from build123d import *

# Parameters (mm, degrees)
SKETCH1_W           = 22
SKETCH1_H           = 31.5
BOSS_EXTRUDE1_DEPTH = 20
SKETCH2_R           = 5.4
CUT_EXTRUDE1_DEPTH  = 20
SKETCH3_R           = 1.5
CUT_EXTRUDE2_DEPTH  = 20
SKETCH4_W           = 22
SKETCH4_H           = 20
SKETCH4_R           = 1.5
BOSS_EXTRUDE2_DEPTH = 0.4
SKETCH5_R           = 44.087047381
CUT_EXTRUDE3_DEPTH  = 0.4
FILLET2_R           = 1
SKETCH6_R           = 1.6
BOSS_EXTRUDE3_DEPTH = 2


with BuildPart() as part:
    # Sketch1 → Boss-Extrude1 (new body)
    with BuildSketch(Plane.XY):
        Polygon((22, 2), (24, 2), (24, -33.5), (-2, -33.5), (-2, 2), align=None)
        with Locations((11, -15.75)):
            Rectangle(SKETCH1_W, SKETCH1_H, mode=Mode.SUBTRACT)
    extrude(amount=BOSS_EXTRUDE1_DEPTH)

    # Sketch2 → Cut-Extrude1 (cut)
    with BuildSketch(Plane(origin=(0, 2, 0), x_dir=(1, 0, 0), z_dir=(0, 1, 0))):
        with Locations((11, -10)):
            Circle(SKETCH2_R)
    extrude(amount=-CUT_EXTRUDE1_DEPTH, mode=Mode.SUBTRACT)

    # Sketch3 → Cut-Extrude2 (cut)
    with BuildSketch(Plane(origin=(0, -33.5, 0), x_dir=(-1, 0, 0), z_dir=(0, -1, 0))):
        with Locations((-11, -10)):
            Circle(SKETCH3_R)
    extrude(amount=-CUT_EXTRUDE2_DEPTH, mode=Mode.SUBTRACT)

    # Sketch4 → Boss-Extrude2 (add)
    with BuildSketch(Plane(origin=(0, -31.5, 0), x_dir=(1, 0, 0), z_dir=(0, 1, 0))):
        with Locations((11, -10)):
            Rectangle(SKETCH4_W, SKETCH4_H)
        with Locations((11, -10)):
            Circle(SKETCH4_R, mode=Mode.SUBTRACT)
    extrude(amount=BOSS_EXTRUDE2_DEPTH)

    # Sketch5 → Cut-Extrude3 (cut)
    with BuildSketch(Plane(origin=(0, -33.5, 0), x_dir=(-1, 0, 0), z_dir=(0, -1, 0))):
        with Locations((-11, -10)):
            Circle(SKETCH5_R)
    extrude(amount=-CUT_EXTRUDE3_DEPTH, mode=Mode.SUBTRACT)

    # Fillet2
    fillet2_edges = [part.edges().sort_by_distance(p)[0] for p in [
        (24, -33.1, 10),
        (-2, -33.1, 10),
        (-2, 2, 10),
        (24, 2, 10),
    ]]
    fillet(fillet2_edges, radius=FILLET2_R)

    # Sketch6 → Boss-Extrude3 (add)
    with BuildSketch(Plane.XY.offset(20)):
        with BuildLine():
            Line((22, -31.1), (27, -31.1))
            ThreePointArc((27, -31.1), (31, -27.1), (27, -23.1))
            Line((27, -23.1), (22, -23.1))
            Line((22, -23.1), (22, -31.1))
        make_face()
        with Locations((27, -27.1)):
            Circle(SKETCH6_R, mode=Mode.SUBTRACT)
        with BuildLine():
            Line((27, -11.1), (22, -11.1))
            Line((22, -11.1), (22, -3.1))
            Line((22, -3.1), (27, -3.1))
            ThreePointArc((27, -3.1), (31, -7.1), (27, -11.1))
        make_face()
        with Locations((27, -7.1)):
            Circle(SKETCH6_R, mode=Mode.SUBTRACT)
        with BuildLine():
            Line((0, -3.1), (-5, -3.1))
            ThreePointArc((-5, -3.1), (-9, -7.1), (-5, -11.1))
            Line((-5, -11.1), (0, -11.1))
            Line((0, -11.1), (0, -3.1))
        make_face()
        with Locations((-5, -7.1)):
            Circle(SKETCH6_R, mode=Mode.SUBTRACT)
        with BuildLine():
            Line((0, -23.1), (0, -31.1))
            Line((0, -31.1), (-5, -31.1))
            ThreePointArc((-5, -31.1), (-9, -27.1), (-5, -23.1))
            Line((-5, -23.1), (0, -23.1))
        make_face()
        with Locations((-5, -27.1)):
            Circle(SKETCH6_R, mode=Mode.SUBTRACT)
    extrude(amount=-BOSS_EXTRUDE3_DEPTH)


solid = part.part
Geometry check sheet. Reference: the model listing, model coordinates, mm. A direction names the side the tool comes from. Give positions to 0.01 mm unless a question says otherwise; leave off trailing zeros. Order: outer loops, then holes, each group sorted by start corner. A loop starts at its lowest first (then second) coordinate and runs counter-clockwise, first axis right, second up.
1) Cross-section at A-A (y = -15.5). Record the boundary of the cut face in (x, z), then the cut area to 3 significant figures.
Results are:
outline: (-2, 0) - (0, 0) - (0, 20) - (-2, 20) - close; (22, 0) - (24, 0) - (24, 20) - (22, 20) - close
area: 80.0 mm2
2) Tool access check on faces 4 (the flat face through (-4, -11.1, 19)), 5 (the flat face through (25, -3.1, 19)), 6 (the flat face through (-6, -5, 18)). Record the directions out of +Z, -Z, +X, -X, +Y, -Y that give a thin tool (end or side, any length) a straight path to the whole face; none if there is none.
Results are:
face 4: +Z, -Z, -X
face 5: +Z, -Z, +X, +Y
face 6: -Z, -X, +Y, -Y
3) Gauge pin test, flat ends, axial feed: pin 1 (1.6 mm diameter, centred on x = -3.5, z = 19, fed in from -Y); pin 2 (12 mm diameter, centred on x = 25, z = 15, fed in from -Y); pin 3 (5.5 mm diameter, centred on x = -7, y = -8, fed in from -Z); pin 4 (12 mm diameter, centred on x = 9.5, y = -16, fed in from -Z). Record the tip position at first contact, or that the pin passes through.
Results are:
pin 1: stops at y = -31.1
pin 2: stops at y = -33.1
pin 3: stops at z = 18
pin 4: passes through
4) Cross-section at D-D (x = 13.5). Record the boundary of the cut face in (y, z), then the cut area to 3 significant figures.
Results are:
outline: (-33.1, 0) - (-31.1, 0) - (-31.1, 20) - (-33.1, 20) - close; (0, 0) - (2, 0) - (2, 5.21) - (0, 5.21) - close; (0, 14.79) - (2, 14.79) - (2, 20) - (0, 20) - close
area: 60.9 mm2
5) Cross-section at B-B (z = 10). Record the boundary of the cut face in (x, y), then the cut area to 3 significant figures.
Results are:
outline: (-2, -32.1) arc R1 ccw to (-1, -33.1) - (9.5, -33.1) - (9.5, -31.1) - (0, -31.1) - (0, 0) - (5.6, 0) - (5.6, 2) - (-1, 2) arc R1 ccw to (-2, 1) - close; (12.5, -33.1) - (23, -33.1) arc R1 ccw to (24, -32.1) - (24, 1) arc R1 ccw to (23, 2) - (16.4, 2) - (16.4, 0) - (22, 0) - (22, -31.1) - (12.5, -31.1) - close
area: 200 mm2
6) Draft check along Y on faces 1 (the cylindrical face through (10.901, -32.114, 8.503)), 2 (the cylindrical face through (-5.35, -28.66, 19.01)), 3 (the cylindrical face through (-1.715, -32.799, 10.14)). Enter one of: released by +Y, released by -Y, zero draft, split by the parting line, or undercut.
Results are:
face 1: zero draft
face 2: undercut
face 3: released by -Y
7) Cross-section at C-C (y = -7.1). Record the boundary of the cut face in (x, z).
Results are:
outline: (-9, 18) - (-6.6, 18) - (-6.6, 20) - (-9, 20) - close; (-3.4, 18) - (-2, 18) - (-2, 0) - (0, 0) - (0, 20) - (-3.4, 20) - close; (22, 0) - (24, 0) - (24, 18) - (25.4, 18) - (25.4, 20) - (22, 20) - close; (28.6, 18) - (31, 18) - (31, 20) - (28.6, 20) - close
8) Material ranges on probe 1 along Y at (x, z) = (-5, 18.55); probe 2 along X at (y, z) = (-23, 17); probe 3 along Y at (x, z) = (0.5, 3.5), recorded low to high.
Results are:
probe 1: y = -31.1 to -28.7, -25.5 to -23.1, -11.1 to -8.7, -5.5 to -3.1
probe 2: x = -2 to 0, 22 to 24
probe 3: y = -33.1 to -31.1, 0 to 2
